```python
from build123d import *

# Parameters (mm, degrees)
SKETCH2_R                       = 14.5
BOSS_EXTRUDE1_DEPTH             = 11
SKETCH4_W                       = 8
SKETCH4_H                       = 4
BOSS_EXTRUDE2_DEPTH             = 8
M3_CLEARANCE_HOLE1_D            = 3.4
MIRROR2_COPY_1_SKETCH_W         = 8
MIRROR2_COPY_1_SKETCH_H         = 4
MIRROR2_COPY_1_DEPTH            = 8
MIRROR2_COPY_2_D                = 3.4
CUT_EXTRUDE1_DEPTH              = 2
M3_CLEARANCE_HOLE2_D            = 3.4
CIRPATTERN1_COUNT               = 4
BOSS_EXTRUDE3_REACH             = 53.246
SKETCH11_W                      = 6
SKETCH11_H                      = 4
BOSS_EXTRUDE3_DIRECTION_2_REACH = 53.246


with BuildPart() as part:
    # Sketch2 → Boss-Extrude1 (new, symmetric)
    with BuildSketch(Plane.XY):
        with BuildLine():
            Line((-21.75, 0), (21.75, 0))
            Line((21.75, 0), (21.75, 18.5))
            ThreePointArc((21.75, 18.5), (0, 40.25), (-21.75, 18.5))
            Line((-21.75, 18.5), (-21.75, 0))
        make_face()
        with Locations((0, 18.5)):
            Circle(SKETCH2_R, mode=Mode.SUBTRACT)
    extrude(amount=BOSS_EXTRUDE1_DEPTH, both=True)

    # Sketch4 → Boss-Extrude2 (add)
    with BuildSketch(Plane.ZY.offset(21.75)):
        with Locations((-7, 2)):
            Rectangle(SKETCH4_W, SKETCH4_H)
    boss_extrude2 = extrude(amount=BOSS_EXTRUDE2_DEPTH)

    # M3 Clearance Hole1 (through all)
    with Locations(Plane(origin=(0, 4, 0), x_dir=(1, 0, 0), z_dir=(0, 1, 0))):
        with Locations((-25.75, 7)):
            m3_clearance_hole1 = Hole(M3_CLEARANCE_HOLE1_D / 2)

    # Mirror1: Boss-Extrude2, M3 Clearance Hole1 across plane
    add(boss_extrude2.mirror(Plane.XY))
    add(m3_clearance_hole1.mirror(Plane.XY), mode=Mode.SUBTRACT)

    # Mirror2: Boss-Extrude2, M3 Clearance Hole1 across plane
    add(boss_extrude2.mirror(Plane(origin=(0, 0, 0), x_dir=(0, 0, 1), z_dir=(1, 0, 0))))
    add(m3_clearance_hole1.mirror(Plane(origin=(0, 0, 0), x_dir=(0, 0, 1), z_dir=(1, 0, 0))), mode=Mode.SUBTRACT)

    # Mirror2 copy 1 sketch → Mirror2 copy 1 (add)
    with BuildSketch(Plane(origin=(21.75, 0, 0), x_dir=(0, 0, -1), z_dir=(1, 0, 0))):
        with Locations((-7, 2)):
            Rectangle(MIRROR2_COPY_1_SKETCH_W, MIRROR2_COPY_1_SKETCH_H)
    extrude(amount=MIRROR2_COPY_1_DEPTH)

    # Mirror2 copy 2 (through all)
    with Locations(Plane(origin=(0, 4, 0), x_dir=(-1, 0, 0), z_dir=(0, 1, 0))):
        with Locations((-25.75, 7)):
            Hole(MIRROR2_COPY_2_D / 2)

    # Sketch8 → Cut-Extrude1 (cut)
    with BuildSketch(Plane(origin=(0, 0, -11), x_dir=(-1, 0, 0), z_dir=(0, 0, -1))):
        with BuildLine():
            Line((-14.318912319, 27.338834765), (-12.620179844, 25.64010229))
            ThreePointArc((-12.620179844, 25.64010229), (-10.253048327, 28.753048327), (-7.14010229, 31.120179844))
            Line((-7.14010229, 31.120179844), (-8.838834765, 32.818912319))
            ThreePointArc((-8.838834765, 32.818912319), (-14.318912319, 32.818912319), (-14.318912319, 27.338834765))
        make_face()
    cut_extrude1 = extrude(amount=-CUT_EXTRUDE1_DEPTH, mode=Mode.SUBTRACT)

    # M3 Clearance Hole2 (through all)
    with Locations(Plane(origin=(0, 0, -9), x_dir=(-1, 0, 0), z_dir=(0, 0, -1))):
        with Locations((-11.578873542, 30.078873542)):
            m3_clearance_hole2 = Hole(M3_CLEARANCE_HOLE2_D / 2)

    # CirPattern1: Cut-Extrude1, M3 Clearance Hole2 ×4 about axis
    cirpattern1_axis = Axis((0, 18.5, 0), (0, 0, 1))
    add([cut_extrude1.rotate(cirpattern1_axis, i * 360 / CIRPATTERN1_COUNT) for i in range(1, CIRPATTERN1_COUNT)], mode=Mode.SUBTRACT)
    add([m3_clearance_hole2.rotate(cirpattern1_axis, i * 360 / CIRPATTERN1_COUNT) for i in range(1, CIRPATTERN1_COUNT)], mode=Mode.SUBTRACT)

    # Boss-Extrude3: up to this face of the body (flat: up to its plane)
    boss_extrude3_end = Plane(part.part.faces().sort_by_distance((29.75, 2, 7))[0])
    # Sketch11 → Boss-Extrude3 (add, up to the picked face)
    with BuildSketch(Plane(origin=(0, 0, 0), x_dir=(0, 0, -1), z_dir=(1, 0, 0)), mode=Mode.PRIVATE) as boss_extrude3_sk1:
        with Locations((0, 2)):
            Rectangle(SKETCH11_W, SKETCH11_H)
    boss_extrude3_tool1 = split(extrude(boss_extrude3_sk1.sketch, amount=BOSS_EXTRUDE3_REACH, mode=Mode.PRIVATE), bisect_by=boss_extrude3_end, keep=Keep.BOTH, mode=Mode.PRIVATE)
    add(boss_extrude3_tool1.solids().sort_by(Axis((0, 2, 0), (1, 0, 0)))[0])

    # Boss-Extrude3 direction 2: up to this face of the body (flat: up to its plane)
    boss_extrude3_direction_2_end = Plane(part.part.faces().sort_by_distance((-29.75, 2, 7))[0])
    # Sketch11 → Boss-Extrude3 direction 2 (add, up to the picked face)
    with BuildSketch(Plane(origin=(0, 0, 0), x_dir=(0, 0, -1), z_dir=(1, 0, 0)), mode=Mode.PRIVATE) as boss_extrude3_direction_2_sk1:
        with Locations((0, 2)):
            Rectangle(SKETCH11_W, SKETCH11_H)
    boss_extrude3_direction_2_tool1 = split(extrude(boss_extrude3_direction_2_sk1.sketch, amount=-BOSS_EXTRUDE3_DIRECTION_2_REACH, mode=Mode.PRIVATE), bisect_by=boss_extrude3_direction_2_end, keep=Keep.BOTH, mode=Mode.PRIVATE)
    add(boss_extrude3_direction_2_tool1.solids().sort_by(Axis((0, 2, 0), (-1, 0, 0)))[0])


solid = part.part
```
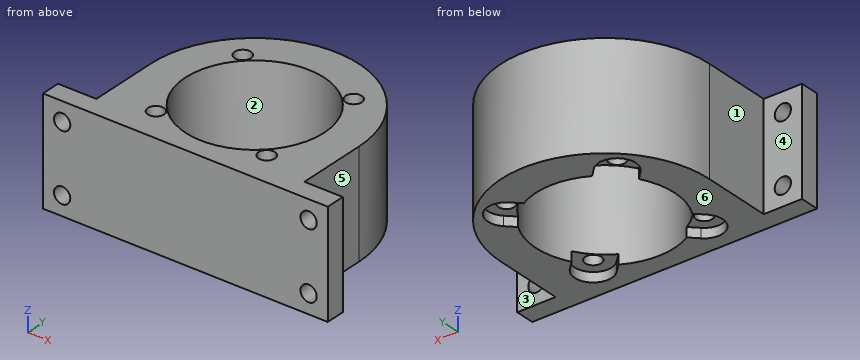
Verification items for the finished model (mm, model axes). Face numbers are marked on the shaded views. A direction names the side the tool comes from. Give positions to 0.01 mm unless a question says otherwise; leave off trailing zeros. Order: outer loops, then holes, each group sorted by start corner. A loop starts at its lowest first (then second) coordinate and runs counter-clockwise, first axis right, second up. Notation, with made-up numbers: (49.5, -34) -> (73.5, -34) arc R16 ccw to (73.5, -5) -> close; hole circle Ø5 at (-12, -22). An arc over 180 degrees is marked (long way). Use a Markdown table: item, result.
1) Material ranges on probe 1 along Z at (x, y) = (-25.75, 2.95); probe 2 along Y at (x, z) = (-12.5, 2.5); probe 3 along X at (y, z) = (18, 7), recorded low to high.
Results:
| item | result |
|---|---|
| probe 1 | -11 to -8.7, -5.3 to 5.3, 8.7 to 11 |
| probe 2 | 0 to 5.49, 8.35 to 11.15, 25.85 to 28.65, 31.51 to 36.3 |
| probe 3 | -21.75 to -14.49, 14.49 to 21.75 |
2) Section check C-C, the plane x = 0. Record the boundary of the cut face in (y, z), then the cut area to 4 significant figures.
Results:
| item | result |
|---|---|
| outline | (0, -11) -> (4, -11) -> (4, 11) -> (0, 11) -> close; (33, -11) -> (40.25, -11) -> (40.25, 11) -> (33, 11) -> close |
| area | 247.5 mm² |
3) Tool access check on the marked faces 4, 5 and 6. Record the directions out of +Z, -Z, +X, -X, +Y, -Y that give a thin tool (end or side, any length) a straight path to the whole face; none if there is none.
Results:
| item | result |
|---|---|
| face 4 | +Z, -Z, -X, +Y |
| face 5 | +Z, -Z, +X, +Y |
| face 6 | -Z, +X, -X, +Y, -Y |
4) Mould release check, pull along Y, two halves, no side actions. Record for the marked faces 1, 2 and 3: pulls with the +Y half, pulls with the -Y half, needs draft (parallel to the pull), parting line crosses it, or undercut.
Results:
| item | result |
|---|---|
| face 1 | needs draft |
| face 2 | undercut |
| face 3 | pulls with the +Y half |
5) Section check D-D, the plane z = 0.5. Record the boundary of the cut face in (x, y), then the cut area to 3 significant figures.
Results:
| item | result |
|---|---|
| outline | (-29.75, 0) -> (29.75, 0) -> (29.75, 4) -> (21.75, 4) -> (21.75, 18.5) arc R21.75 ccw to (-21.75, 18.5) -> (-21.75, 4) -> (-29.75, 4) -> close; hole circle Ø29 at (0, 18.5); hole circle Ø3.4 at (-11.58, 6.92); hole circle Ø3.4 at (-11.58, 30.08); hole circle Ø3.4 at (11.58, 6.92); hole circle Ø3.4 at (11.58, 30.08) |
| area | 915 mm² |
6) Section check B-B, the plane z = 7. Record the boundary of the cut face in (x, y).
Results:
| item | result |
|---|---|
| outline | (-29.75, 0) -> (-27.45, 0) -> (-27.45, 4) -> (-29.75, 4) -> close; (-24.05, 0) -> (24.05, 0) -> (24.05, 4) -> (21.75, 4) -> (21.75, 18.5) arc R21.75 ccw to (-21.75, 18.5) -> (-21.75, 4) -> (-24.05, 4) -> close; (27.45, 0) -> (29.75, 0) -> (29.75, 4) -> (27.45, 4) -> close; hole circle Ø29 at (0, 18.5); hole circle Ø3.4 at (-11.58, 6.92); hole circle Ø3.4 at (-11.58, 30.08); hole circle Ø3.4 at (11.58, 6.92); hole circle Ø3.4 at (11.58, 30.08) |
7) Depth check by flat-ended pin: pin 1 Ø2.5 at (x, y) = (-12.5, 30.5) entering from -Z; pin 2 Ø10 at (x, z) = (6.5, 5.5) entering from +Y; pin 3 Ø4.5 at (y, z) = (13.5, 4.5) entering from +X. Enter the tip coordinate at first touch or a pass-through.
Results:
| item | result |
|---|---|
| pin 1 | z = -9 |
| pin 2 | y = 40.2 |
| pin 3 | x = 21.75 |
8) Section check A-A, the plane x = 25.75. Record the boundary of the cut face in (y, z), then the cut area to 3 significant figures.
Results:
| item | result |
|---|---|
| outline | (0, -11) -> (4, -11) -> (4, -8.7) -> (0, -8.7) -> close; (0, -5.3) -> (4, -5.3) -> (4, 5.3) -> (0, 5.3) -> close; (0, 8.7) -> (4, 8.7) -> (4, 11) -> (0, 11) -> close |
| area | 60.8 mm² |
